from build123d import *

# Parameters (mm, degrees)
SKETCH1_R           = 3.25
BOSS_EXTRUDE1_DEPTH = 49
FILLET1_R           = 4
SKETCH2_R           = 5.5
CUT_EXTRUDE1_DEPTH  = 33
SKETCH3_R           = 1.2
CUT_EXTRUDE2_DEPTH  = 54.875656369


with BuildPart() as part:
    # Sketch1 → Boss-Extrude1 (new body)
    with BuildSketch(Plane(origin=(0, 0, 0), x_dir=(1, 0, 0), z_dir=(0, 1, 0))):
        Polygon((-5.320759509, 8), (-22.469015665, -7.56), (22.469015665, -7.56), (5.320759509, 8), align=None)
        with Locations(Location((0, 0, 0), (0, 0, 270))):
            Circle(SKETCH1_R, mode=Mode.SUBTRACT)
    extrude(amount=BOSS_EXTRUDE1_DEPTH)

    # Fillet1
    fillet1_edges = [part.edges().sort_by_distance(p)[0] for p in [
        (5.320759509, 24.5, -8),
        (22.469015665, 24.5, 7.56),
        (-22.469015665, 24.5, 7.56),
        (-5.320759509, 24.5, -8),
    ]]
    fillet(fillet1_edges, radius=FILLET1_R)

    # Sketch2 → Cut-Extrude1 (cut)
    with BuildSketch(Plane(origin=(0, 49, 0), x_dir=(1, 0, 0), z_dir=(0, 1, 0))):
        with Locations(Location((0, 0, 0), (0, 0, 270))):
            Circle(SKETCH2_R)
    extrude(amount=-CUT_EXTRUDE1_DEPTH, mode=Mode.SUBTRACT)

    # Sketch3 → Cut-Extrude2 (cut, through all)
    with BuildSketch(Plane.XY.offset(7.56)):
        with Locations((-7.5, 40)):
            Circle(SKETCH3_R)
        with Locations((7.5, 40)):
            Circle(SKETCH3_R)
        with Locations((7.5, 30)):
            Circle(SKETCH3_R)
        with Locations((-7.5, 30)):
            Circle(SKETCH3_R)
    extrude(amount=-CUT_EXTRUDE2_DEPTH, mode=Mode.SUBTRACT)


solid = part.part
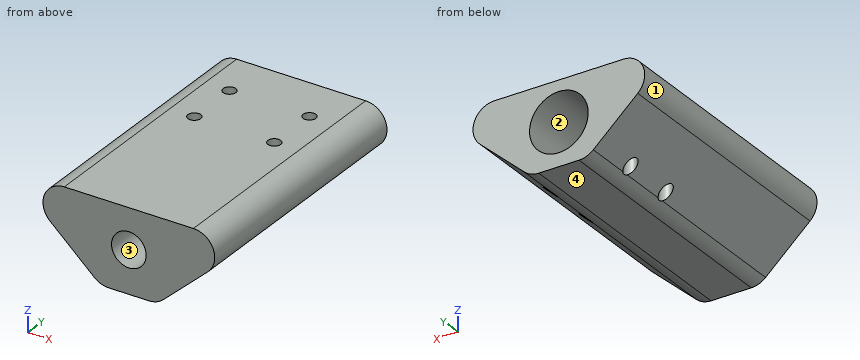
Geometry: final body of the model. Coordinates: model frame, mm. Face numbers are marked on the shaded views. Coordinates: 2 decimals unless noted, no trailing zeros. Order: outer loops, then holes, each group sorted by start corner. A loop starts at its lowest first (then second) coordinate and runs counter-clockwise, first axis right, second up.
1) Section A-A (y = 22.5). Return loops of the section in (x, z), then the cut area to 3 significant figures.
Result sheet:
outline: (-14.8, 0.6) - (-6.46, -6.96) arc R4 ccw to (-3.78, -8) - (3.78, -8) arc R4 ccw to (6.46, -6.96) - (14.8, 0.6) arc R4 ccw to (12.11, 7.56) - (-12.11, 7.56) arc R4 ccw to start; hole circle Ø11 at (0, 0)
area: 292 mm2
2) Ray query, probe 1 along Y at (x, z) = (-7.5, 4.25); probe 2 along X at (y, z) = (39, 0); probe 3 along Z at (x, y) = (0, 3). Return the intervals inside material, ascending.
Result sheet:
probe 1: y = 0 to 28.8, 31.2 to 38.8, 41.2 to 49
probe 2: x = -14.14 to -8.16, -6.84 to -5.5, 5.5 to 6.84, 8.16 to 14.14
probe 3: z = -8 to -3.25, 3.25 to 7.56
3) First-contact query: P1, Ø3, axis at x = 7.5, y = 30, coming from the -Z side; P2, Ø6, axis at y = 17, z = -1.5, coming from the -X side; P3, Ø1, axis at y = 29.5, z = -5.5, coming from the +X side. Flat tips, straight axial feed; report the tip coordinate or a pass-through.
Result sheet:
P1: stops at z = -7.33
P2: stops at x = -15.54
P3: stops at x = 8.63
4) Section C-C (z = -1). Return loops of the section in (x, y), then the cut area to 3 significant figures.
Result sheet:
outline: (-13.04, 0) - (-3.09, 0) - (-3.09, 16) - (-5.41, 16) - (-5.41, 49) - (-13.04, 49) - close; (3.09, 0) - (13.04, 0) - (13.04, 49) - (5.41, 49) - (5.41, 16) - (3.09, 16) - close; hole circle Ø2.4 at (-7.5, 30); hole circle Ø2.4 at (-7.5, 40); hole circle Ø2.4 at (7.5, 30); hole circle Ø2.4 at (7.5, 40)
area: 803 mm2
5) Section B-B (x = 0). Return loops of the section in (y, z), then the cut area to 3 significant figures.
Result sheet:
outline: (0, -8) - (49, -8) - (49, -5.5) - (16, -5.5) - (16, -3.25) - (0, -3.25) - close; (0, 3.25) - (16, 3.25) - (16, 5.5) - (49, 5.5) - (49, 7.56) - (0, 7.56) - close
area: 295 mm2
6) Draft query along X for the marked faces 1, 2, 3 and 4. Return one class per face: released by +X, released by -X, zero draft, split by the parting line, or undercut.
Result sheet:
face 1: released by -X
face 2: undercut
face 3: undercut
face 4: zero draft
7) Section D-D (y = 40). Return loops of the section in (x, z).
Result sheet:
outline: (-14.8, 0.6) - (-8.7, -4.93) - (-8.7, 7.56) - (-12.11, 7.56) arc R4 ccw to start; (-6.3, -7.1) arc R4 ccw to (-3.78, -8) - (3.78, -8) arc R4 ccw to (6.3, -7.1) - (6.3, 7.56) - (-6.3, 7.56) - close; (8.7, -4.93) - (14.8, 0.6) arc R4 ccw to (12.11, 7.56) - (8.7, 7.56) - close; hole circle Ø11 at (0, 0)
